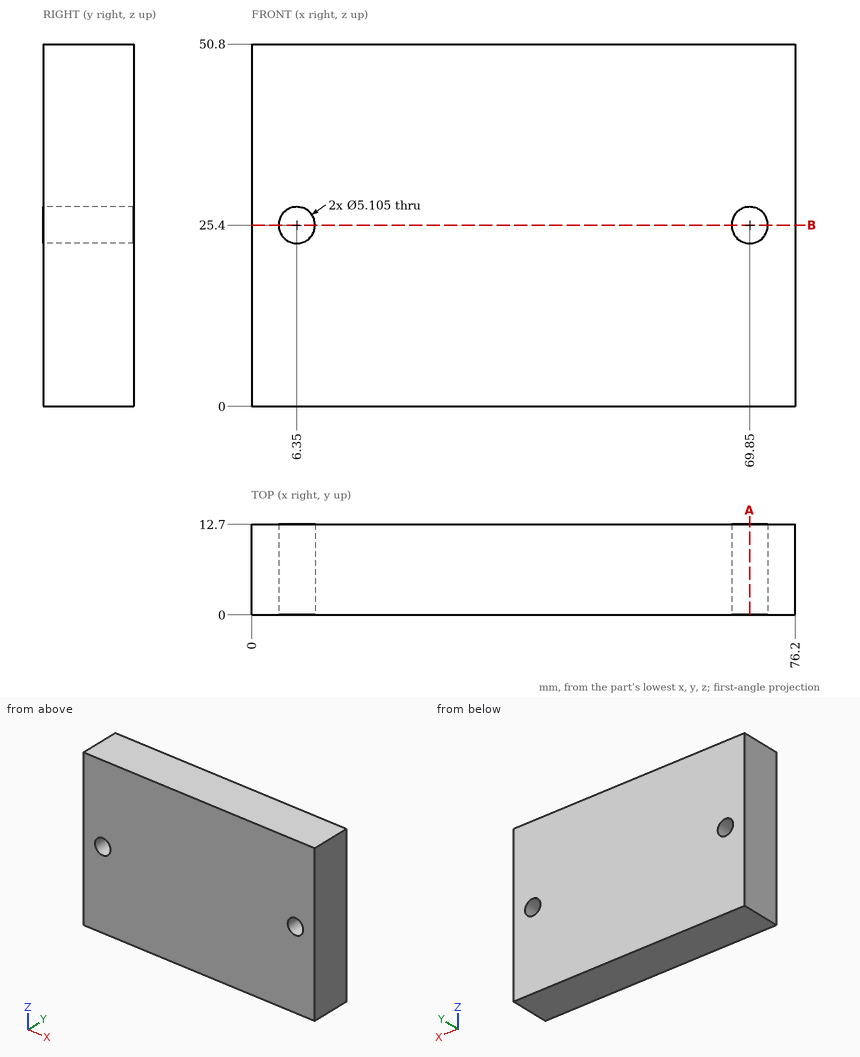
Part print with two shaded views. Sizes in mm from the minimum x, y, z corner. Round coordinates to 2 decimals unless told otherwise and drop trailing zeros. Loops run counter-clockwise (first coordinate to the right, second up) from the corner with the lowest first, then second, coordinate; pieces in that order, holes last.
1. Slice it at A-A (x = 69.85). Give the cut face in (y, z), and give its area (3 significant figures).
Solutions:
outline: (0, 0) - (12.7, 0) - (12.7, 22.85) - (0, 22.85) - close; (0, 27.95) - (12.7, 27.95) - (12.7, 50.8) - (0, 50.8) - close
area: 580 mm2
2. Slice it at B-B (z = 25.4). Give the cut face in (x, y).
Solutions:
outline: (0, 0) - (3.8, 0) - (3.8, 12.7) - (0, 12.7) - close; (8.9, 0) - (67.3, 0) - (67.3, 12.7) - (8.9, 12.7) - close; (72.4, 0) - (76.2, 0) - (76.2, 12.7) - (72.4, 12.7) - close
3. Drill centre lines: line 1 along X through (y, z) = (10, 25.4); line 2 along Z through (x, y) = (6.35, 5). Where is each one in solid material? Low to high.
Solutions:
line 1: x = 0 to 3.8, 8.9 to 67.3, 72.4 to 76.2
line 2: z = 0 to 22.85, 27.95 to 50.8
